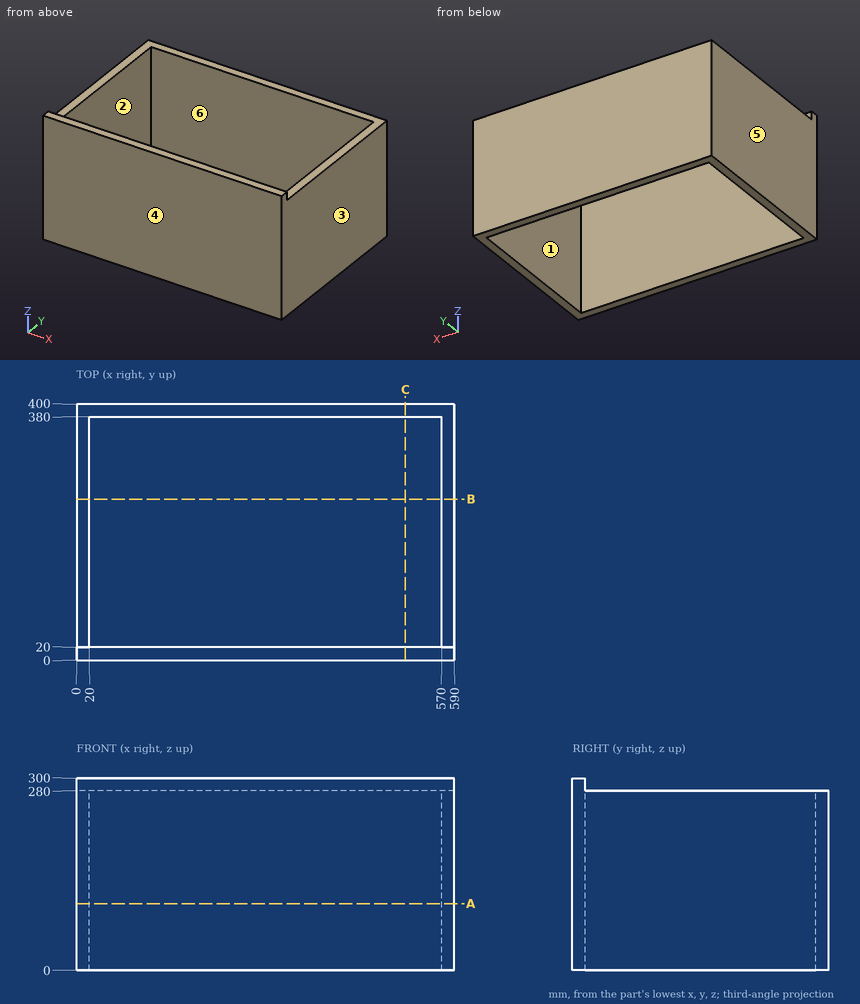
Drawing for the job (mm, zero at the part's lowest x, y, z). A direction names the side the tool comes from. Round coordinates to 2 decimals unless told otherwise and drop trailing zeros. Loops run counter-clockwise (first coordinate to the right, second up) from the corner with the lowest first, then second, coordinate; pieces in that order, holes last. Notation, with made-up numbers: M 84,56.25 L 119,56.25 A16 ccw 119,71.25 Z; hole C -24,-30.75 d2. An arc over 180 degrees is marked long. Use a Markdown table: item, result. Add a question column.
(1) Cut at C-C (x = 513.5). Give the cut face in (y, z), and give its area (3 significant figures).
(2) Pull direction Y, two halves, no side cores. Call the marked faces 1, 2, 3 and 4: +Y half, -Y half, draft (parallel to the pull), parting line (faces both ways), or undercut.
(3) Flat gauge pin, fed straight in: pin 1 (1.5 mm diameter, centred on y = 348, z = 197, fed in from -X). Where does the tip first touch, or does it go through?
(4) Which spindle directions (+Z, -Z, +X, -X, +Y, -Y) get a long thin tool onto all of the face, cutting with end or side? Do the marked faces 5 and 6. Say none if no direction does.
(5) Cut at B-B (y = 251.5). Give the cut face in (x, z).
(6) Cut at A-A (z = 104). Give the cut face in (x, y), and give its area (3 significant figures).
(7) Drill centre lines: line 1 (Y direction, x = 438, z = 228.5); line 2 (X direction, y = 75, z = 36). Where is each one in solid material? Low to high.
Geometry says:
| question | item | result |
|---|---|---|
| 1 | outline | M 0,0 L 20,0 L 20,300 L 0,300 Z; M 380,0 L 400,0 L 400,280 L 380,280 Z |
| 1 | area | 11,600 mm² |
| 2 | face 1 | undercut |
| 2 | face 2 | undercut |
| 2 | face 3 | draft |
| 2 | face 4 | -Y half |
| 3 | pin 1 | stops at x = 0 |
| 4 | face 5 | +Z, -Z, -X, +Y, -Y |
| 4 | face 6 | +Z, -Z |
| 5 | outline | M 0,0 L 20,0 L 20,280 L 0,280 Z; M 570,0 L 590,0 L 590,280 L 570,280 Z |
| 6 | outline | M 0,0 L 590,0 L 590,400 L 0,400 Z; hole M 20,20 L 570,20 L 570,380 L 20,380 Z |
| 6 | area | 38,000 mm² |
| 7 | line 1 | y = 0 to 20, 380 to 400 |
| 7 | line 2 | x = 0 to 20, 570 to 590 |
